Work out the finished part from the listing and answer in its coordinate system (mm). A direction names the side the tool comes from. Coordinates: 2 decimals unless noted, no trailing zeros. Order: outer loops, then holes, each group sorted by start corner. A loop starts at its lowest first (then second) coordinate and runs counter-clockwise, first axis right, second up.
```python
from build123d import *

# Parameters (mm, degrees)
F0_W     = 139.7
F0_H     = 76.2
F0_W_2   = 19.05
F1_DEPTH = 19.05


with BuildPart() as f1:
    # F0 (on Front) → F1 (new body)
    with BuildSketch(Plane.XZ):
        with Locations((0, 209.55)):
            Rectangle(F0_W, F0_H)
        Polygon((69.85, 171.45), (-69.85, 171.45), (-69.85, 95.25), (-69.85, -82.55), (-69.85, -158.75), (69.85, -158.75), (69.85, -82.55), (69.85, 95.25), align=None)
        with Locations((-79.375, 133.35)):
            Rectangle(F0_W_2, F0_H)
        with Locations((79.375, 133.35)):
            Rectangle(F0_W_2, F0_H)
        with Locations((-79.375, -120.65)):
            Rectangle(F0_W_2, F0_H)
        with Locations((79.375, -120.65)):
            Rectangle(F0_W_2, F0_H)
        with Locations((0, -196.85)):
            Rectangle(F0_W, F0_H)
    extrude(amount=F1_DEPTH)


solid = f1.part
```
1. Flat-ended cylindrical pins translate along their axes: pin 1 (5.5 mm diameter, centred on x = -82.5, y = -13.5, fed in from +Z); pin 2 (9.5 mm diameter, centred on y = -12, z = -183.5, fed in from +X); pin 3 (5.5 mm diameter, centred on y = -10.5, z = -189, fed in from -X). Find the tip coordinate at first contact, or state that the pin passes through.
2. The part is cut by section C-C (z = 89.5). Determine the outline of the cut face in (x, y).
3. The part is cut by section A-A (x = 74). Determine the outline of the cut face in (y, z).
4. The part is cut by section B-B (y = -15.25). Determine the outline of the cut face in (x, z).
5. The mould has two halves that part along Z. Classify faces 4 (the flat face through (-1, -9, -234.95)), 5 (the flat face through (69.85, -9, 5)), 6 (the flat face through (-88.9, -9, -121)), 7 (the flat face through (-80, -9, -82.55)): released by +Z, released by -Z, zero draft, split by the parting line, or undercut.
6. For faces 1 (the flat face through (79, -9, 95.25)), 2 (the flat face through (-80, -9, 171.45)), 3 (the flat face through (79, -9, 171.45)), determine the directions among +Z, -Z, +X, -X, +Y, -Y from which every point of the face is accessible in a straight line to the end or side of a thin tool.
7. Consider probe 1 along X at (y, z) = (-2, 227.5); probe 2 along Z at (x, y) = (80, -11.25). Determine where each line is inside the solid, lowest interval first.
Worked out:
1. pin 1: stops at z = 171.45
1. pin 2: stops at x = 69.85
1. pin 3: stops at x = -69.85
2. outline: (-69.85, -19.05) - (69.85, -19.05) - (69.85, 0) - (-69.85, 0) - close
3. outline: (-19.05, -158.75) - (0, -158.75) - (0, -82.55) - (-19.05, -82.55) - close; (-19.05, 95.25) - (0, 95.25) - (0, 171.45) - (-19.05, 171.45) - close
4. outline: (-88.9, -158.75) - (-69.85, -158.75) - (-69.85, -234.95) - (69.85, -234.95) - (69.85, -158.75) - (88.9, -158.75) - (88.9, -82.55) - (69.85, -82.55) - (69.85, 95.25) - (88.9, 95.25) - (88.9, 171.45) - (69.85, 171.45) - (69.85, 247.65) - (-69.85, 247.65) - (-69.85, 171.45) - (-88.9, 171.45) - (-88.9, 95.25) - (-69.85, 95.25) - (-69.85, -82.55) - (-88.9, -82.55) - close
5. face 4: released by -Z
5. face 5: undercut
5. face 6: zero draft
5. face 7: undercut
6. face 1: +X, +Y, -Y
6. face 2: +Z, -X, +Y, -Y
6. face 3: +Z, +X, +Y, -Y
7. probe 1: x = -69.85 to 69.85
7. probe 2: z = -158.75 to -82.55, 95.25 to 171.45
